The listing builds one solid part. Answer for the finished solid, in the listing's coordinates (mm). A direction names the side the tool comes from. Round coordinates to 2 decimals unless told otherwise and drop trailing zeros. Write each loop counter-clockwise with the first axis right and the second up, starting at its lowest first coordinate (ties: lowest second). Pieces come first, ordered by that corner, then holes. Notation, with made-up numbers: (68, 52) -> (85, 52) arc R18 cw to (85, 58) -> close; hole circle Ø4 at (-27.75, 36.5). An arc over 180 degrees is marked (long way). Write each question's results on one line, items separated by ' | '. Start each with the question number.
```python
from build123d import *

# Parameters (mm, degrees)
SKETCH1_W                = 8
SKETCH1_H                = 15
BOSS_EXTRUDE1_DEPTH      = 4
CUT_EXTRUDE1_DEPTH       = 6
M3_CLEARANCE_HOLE2_D     = 3.2
M3_CLEARANCE_HOLE2_DEPTH = 12
SKETCH9_R                = 0.85
BOSS_EXTRUDE2_DEPTH      = 1
SKETCH12_W               = 8
SKETCH12_H               = 6
BOSS_EXTRUDE3_DEPTH      = 8
M5_CLEARANCE_HOLE1_D     = 5.3
BOSS_EXTRUDE4_START      = -6
SKETCH18_R               = 2.65
BOSS_EXTRUDE4_DEPTH      = 6
BOSS_EXTRUDE5_DEPTH      = 11
FILLET2_R                = 2


with BuildPart() as part:
    # Sketch1 → Boss-Extrude1 (new, symmetric)
    with BuildSketch(Plane.XY):
        Rectangle(SKETCH1_W, SKETCH1_H)
    extrude(amount=BOSS_EXTRUDE1_DEPTH, both=True)

    # Sketch2 → Cut-Extrude1 (cut)
    with BuildSketch(Plane.XY.offset(4)):
        Polygon((-3, 4.5), (3, 4.5), (3, 1.325), (-4, 1.325), (-4, 3.5), (-3, 3.5), align=None)
        Polygon((4, -4.5), (-3, -4.5), (-3, -1.325), (3, -1.325), (3, -2.325), (4, -2.325), align=None)
    extrude(amount=-CUT_EXTRUDE1_DEPTH, mode=Mode.SUBTRACT)

    # M3 Clearance Hole2
    with Locations(Plane(origin=(0, 7.5, 0), x_dir=(1, 0, 0), z_dir=(0, 1, 0))):
        with Locations((0, -1)):
            Hole(M3_CLEARANCE_HOLE2_D / 2, depth=M3_CLEARANCE_HOLE2_DEPTH)

    # Sketch9 → Boss-Extrude2 (add)
    with BuildSketch(Plane.XY.offset(4)):
        with Locations(Location((0, 6, 0), (0, 0, 180))):
            Circle(SKETCH9_R)
        with Locations(Location((0, -6, 0), (0, 0, 180))):
            Circle(SKETCH9_R)
    extrude(amount=BOSS_EXTRUDE2_DEPTH)

    # Sketch12 → Boss-Extrude3 (add)
    with BuildSketch(Plane(origin=(0, 0, -4), x_dir=(-1, 0, 0), z_dir=(0, 0, -1))):
        with Locations((0, 4.5)):
            Rectangle(SKETCH12_W, SKETCH12_H)
    extrude(amount=BOSS_EXTRUDE3_DEPTH)

    # M5 Clearance Hole1 (through all)
    with Locations(Plane(origin=(0, 7.5, 0), x_dir=(1, 0, 0), z_dir=(0, 1, 0))):
        with Locations((0, 8)):
            Hole(M5_CLEARANCE_HOLE1_D / 2)

    # Sketch18 → Boss-Extrude4 (add)
    with BuildSketch(Plane(origin=(0, 7.5, 0), x_dir=(1, 0, 0), z_dir=(0, 1, 0)).offset(BOSS_EXTRUDE4_START)):
        Polygon((4.618802154, 8), (2.309401077, 12), (-2.309401077, 12), (-4.618802154, 8), (-2.309401077, 4), (2.309401077, 4), align=None)
        with Locations(Location((0, 8, 0), (0, 0, 270))):
            Circle(SKETCH18_R, mode=Mode.SUBTRACT)
    extrude(amount=BOSS_EXTRUDE4_DEPTH)

    # Sketch19 → Boss-Extrude5 (add)
    with BuildSketch(Plane(origin=(0, 7.5, 0), x_dir=(1, 0, 0), z_dir=(0, 1, 0))):
        Polygon((4, 2.92820323), (6.92820323, 8), (3.464101615, 14), (-3.464101615, 14), (-6.92820323, 8), (-4, 2.92820323), (-4, 6.92820323), (-4.618802154, 8), (-4, 9.07179677), (-4, 12), (-2.309401077, 12), (2.309401077, 12), (4, 12), (4, 9.07179677), (4.618802154, 8), (4, 6.92820323), align=None)
        Polygon((2.309401077, 12), (4, 9.07179677), (4, 12), align=None)
        Polygon((-4, 9.07179677), (-2.309401077, 12), (-4, 12), align=None)
        Polygon((3.464101615, 2), (4, 2.92820323), (4, 6.92820323), (2.309401077, 4), (-2.309401077, 4), (-4, 6.92820323), (-4, 2.92820323), (-3.464101615, 2), align=None)
    extrude(amount=-BOSS_EXTRUDE5_DEPTH)

    # Fillet2
    fillet2_edges = [part.edges().sort_by_distance(p)[0] for p in [
        (6.92820323, 2, -8),
        (-4, 2, -2.92820323),
        (-6.92820323, 2, -8),
        (-3.464101615, 2, -14),
        (3.464101615, 2, -14),
        (4, 2, -2.92820323),
    ]]
    fillet(fillet2_edges, radius=FILLET2_R)


solid = part.part
```
Q1. The part is cut by section B-B, the plane y = 6. Write down the section's boundary in (x, z).
Q2. For faces 4 (the cylindrical face through (0.35, 5.98, 2.56)), 5 (the flat face through (3.5, -2.325, 1)), 6 (the flat face through (0, 2, -14)), 7 (the flat face through (3, 3, 1)), 8 (the cylindrical face through (0.57, 4.46, -5.41)), determine the directions among +Z, -Z, +X, -X, +Y, -Y from which every point of the face is accessible in a straight line to the end or side of a thin tool.
Q3. Find the intervals of material crossed by line 1 (Z direction, x = 0, y = 5.2); line 2 (Z direction, x = 0, y = 0.3); line 3 (Y direction, x = 2.5, z = 2.25) (3 decimals), in increasing order.
Q4. The part is cut by section D-D, the plane z = -1.75. Write down the section's boundary in (x, y) (3 decimals).
Q5. Each of these flat-tipped pins is pushed along its axis until it touches: pin 1 (1.6 mm diameter, centred on y = 2, z = -0.5, fed in from -X); pin 2 (5 mm diameter, centred on x = 0.5, y = -2, fed in from +Z); pin 3 (6.5 mm diameter, centred on y = 1.5, z = -2, fed in from +X). Where does it stop, or does it pass through?
Q6. The part is cut by section A-A, the plane z = 1. Write down the section's boundary in (x, y) (3 decimals).
Q7. Determine the mould class of faces 1 (the flat face through (-2, 1.325, 1)), 2 (the cylindrical face through (0.18, 6.83, 4.49)), 3 (the cylindrical face through (0.35, -0.02, 2.56)) for opening direction Y: pulls with the +Y half, pulls with the -Y half, needs draft (parallel to the pull), parting line crosses it, or undercut.
Q8. The part is cut by section C-C, the plane y = 2.25. Write down the section's boundary in (x, z), then the cut area to 3 significant figures.
Answers follow:
1) outline: (-6.35, -9) -> (-4.04, -13) arc R2 ccw to (-2.31, -14) -> (2.31, -14) arc R2 ccw to (4.04, -13) -> (6.35, -9) arc R2 ccw to (6.35, -7) -> (4.27, -3.39) arc R2 cw to (4, -2.39) -> (4, 4) -> (0.85, 4) -> (0.85, 5) -> (-0.85, 5) -> (-0.85, 4) -> (-4, 4) -> (-4, -2.39) arc R2 cw to (-4.27, -3.39) -> (-6.35, -7) arc R2 ccw to start; hole circle Ø5.3 at (0, -8); hole circle Ø3.2 at (0, 1)
2) face 4: +Y | face 5: +Z, +X | face 6: -Z, +X, -X, +Y, -Y | face 7: +Z | face 8: +Y, -Y
3) line 1: -14 to -10.65, -5.35 to -0.6, 2.6 to 5 | line 2: -14 to -12, -4 to -0.6, 2.6 to 4 | line 3: -7.5 to -4.5, -1.325 to 1.325, 4.5 to 7.5
4) outline: (-4, -7.5) -> (4, -7.5) -> (4, -4.5) -> (-3, -4.5) -> (-3, -1.325) -> (3, -1.325) -> (3, -2.325) -> (4, -2.325) -> (4, 7.5) -> (-4, 7.5) -> (-4, 3.5) -> (-3, 3.5) -> (-3, 4.5) -> (3, 4.5) -> (3, 1.325) -> (-4, 1.325) -> close
5) pin 1: x = -4 | pin 2: z = 4 | pin 3: x = 5.34
6) outline: (-4, -7.5) -> (4, -7.5) -> (4, -4.5) -> (-3, -4.5) -> (-3, -1.325) -> (-1.6, -1.325) -> (-1.6, 1.325) -> (-4, 1.325) -> close; (-4, 3.5) -> (-3, 3.5) -> (-3, 4.5) -> (-1.6, 4.5) -> (-1.6, 7.5) -> (-4, 7.5) -> close; (1.6, -1.325) -> (3, -1.325) -> (3, -2.325) -> (4, -2.325) -> (4, 7.5) -> (1.6, 7.5) -> (1.6, 4.5) -> (3, 4.5) -> (3, 1.325) -> (1.6, 1.325) -> close
7) face 1: undercut | face 2: undercut | face 3: needs draft
8) outline: (-6.35, -9) -> (-4.04, -13) arc R2 ccw to (-2.31, -14) -> (2.31, -14) arc R2 ccw to (4.04, -13) -> (6.35, -9) arc R2 ccw to (6.35, -7) -> (4.27, -3.39) arc R2 cw to (4, -2.39) -> (4, 4) -> (3, 4) -> (3, -2) -> (-4, -2) -> (-4, -2.39) arc R2 cw to (-4.27, -3.39) -> (-6.35, -7) arc R2 ccw to start; hole circle Ø5.3 at (0, -8) | area: 108 mm^2
